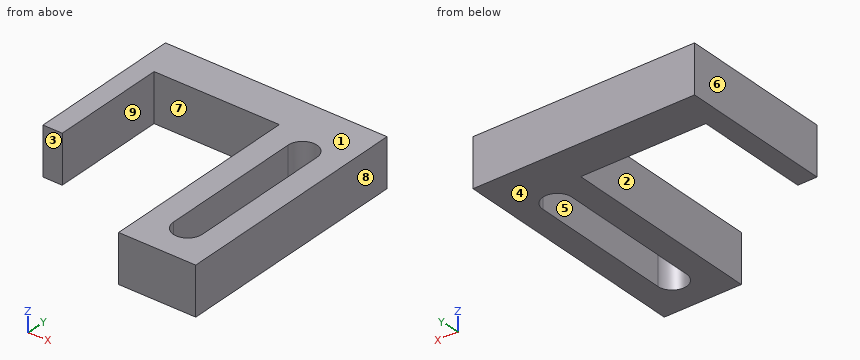
from build123d import *

# Parameters (mm, degrees)
SKETCH1_W           = 8
SKETCH1_H           = 25
BOSS_EXTRUDE6_DEPTH = 2.5
SKETCH8_W           = 15
SKETCH8_H           = 4
BOSS_EXTRUDE7_DEPTH = 5
SKETCH9_W           = 2
SKETCH9_H           = 5
BOSS_EXTRUDE8_DEPTH = 12
CUT_EXTRUDE1_DEPTH  = 6


with BuildPart() as part:
    # Sketch1 → Boss-Extrude6 (new body, symmetric)
    with BuildSketch(Plane.XY):
        Rectangle(SKETCH1_W, SKETCH1_H)
    extrude(amount=BOSS_EXTRUDE6_DEPTH, both=True)

    # Sketch8 → Boss-Extrude7 (add)
    with BuildSketch(Plane.XY.offset(2.5)):
        with Locations((-11.5, 10.5)):
            Rectangle(SKETCH8_W, SKETCH8_H)
    extrude(amount=-BOSS_EXTRUDE7_DEPTH)

    # Sketch9 → Boss-Extrude8 (add)
    with BuildSketch(Plane.XZ.offset(-8.5)):
        with Locations((-18, 0)):
            Rectangle(SKETCH9_W, SKETCH9_H)
    extrude(amount=BOSS_EXTRUDE8_DEPTH)

    # Sketch10 → Cut-Extrude1 (cut, through all)
    with BuildSketch(Plane.XY.offset(2.5)):
        with BuildLine():
            Line((1.5, 6.5), (1.5, -8.5))
            ThreePointArc((1.5, -8.5), (0, -10), (-1.5, -8.5))
            Line((-1.5, -8.5), (-1.5, 6.5))
            ThreePointArc((-1.5, 6.5), (0, 8), (1.5, 6.5))
        make_face()
    extrude(amount=-CUT_EXTRUDE1_DEPTH, mode=Mode.SUBTRACT)


solid = part.part
Input: part model. Units: mm. Frame: model coordinates. Face numbers are marked on the shaded views. A direction names the side the tool comes from. Round coordinates to 2 decimals unless told otherwise and drop trailing zeros. Loops run counter-clockwise (first coordinate to the right, second up) from the corner with the lowest first, then second, coordinate; pieces in that order, holes last. Notation, with made-up numbers: (-4, 13) -> (47, 13) arc R27 cw to (47, 42) -> close; hole circle Ø9 at (46.25, 62.5). An arc over 180 degrees is marked (long way). Answer as a JSON object with one key per item and string values. Group by question number.
1) Draft query along X for the marked faces 6, 7, 8 and 9. Return one class per face: +X half, -X half, draft (parallel to the pull), parting line (faces both ways), or undercut.
2) Section query D-D on z = -1.2. Output: boundary loops of the cut face in (x, y).
3) Section query A-A on y = -6.75. Output: boundary loops of the cut face in (x, z), plus the area to 3 significant figures.
4) Section query C-C on y = 4.75. Output: boundary loops of the cut face in (x, z).
5) Section query B-B on x = 0. Output: boundary loops of the cut face in (y, z).
6) Pin query (flat end, axial travel): pin 1 (0.6 mm diameter, centred on x = -18, z = -1, fed in from -Y); pin 2 (1.5 mm diameter, centred on x = -16, z = 0, fed in from -Y). Return the tip coordinate at first contact, or that it passes through.
7) Reachability of the marked faces 1, 2, 3, 4 and 5 from +Z, -Z, +X, -X, +Y, -Y: full face, straight path, thin tool, end or side. Return the list, or none.
8) Ray query, L1, parallel to X at y = 4, z = 1.95; L2, parallel to X at y = -7.25, z = 0.25; L3, parallel to X at y = 7, z = 0.05. Return the intervals inside material, ascending.
Reply:
{
 "1": {"face 6": "-X half", "face 7": "undercut", "face 8": "+X half", "face 9": "undercut"},
 "2": {"outline": "(-19, -3.5) -> (-17, -3.5) -> (-17, 8.5) -> (-4, 8.5) -> (-4, -12.5) -> (4, -12.5) -> (4, 12.5) -> (-19, 12.5) -> close; hole (-1.5, -8.5) arc R1.5 ccw to (1.5, -8.5) -> (1.5, 6.5) arc R1.5 ccw to (-1.5, 6.5) -> close"},
 "3": {"outline": "(-4, -2.5) -> (-1.5, -2.5) -> (-1.5, 2.5) -> (-4, 2.5) -> close; (1.5, -2.5) -> (4, -2.5) -> (4, 2.5) -> (1.5, 2.5) -> close", "area": "25.0 mm2"},
 "4": {"outline": "(-19, -2.5) -> (-17, -2.5) -> (-17, 2.5) -> (-19, 2.5) -> close; (-4, -2.5) -> (-1.5, -2.5) -> (-1.5, 2.5) -> (-4, 2.5) -> close; (1.5, -2.5) -> (4, -2.5) -> (4, 2.5) -> (1.5, 2.5) -> close"},
 "5": {"outline": "(-12.5, -2.5) -> (-10, -2.5) -> (-10, 2.5) -> (-12.5, 2.5) -> close; (8, -2.5) -> (12.5, -2.5) -> (12.5, 2.5) -> (8, 2.5) -> close"},
 "6": {"pin 1": "stops at y = -3.5", "pin 2": "stops at y = 8.5"},
 "7": {"face 1": "+Z, +X, -X, +Y, -Y", "face 2": "+Z, -Z, -Y", "face 3": "+Z, -Z, -X, -Y", "face 4": "-Z, +X, -X, +Y, -Y", "face 5": "+Z, -Z"},
 "8": {"L1": "x = -19 to -17, -4 to -1.5, 1.5 to 4", "L2": "x = -4 to -1.5, 1.5 to 4", "L3": "x = -19 to -17, -4 to -1.41, 1.41 to 4"}
}
